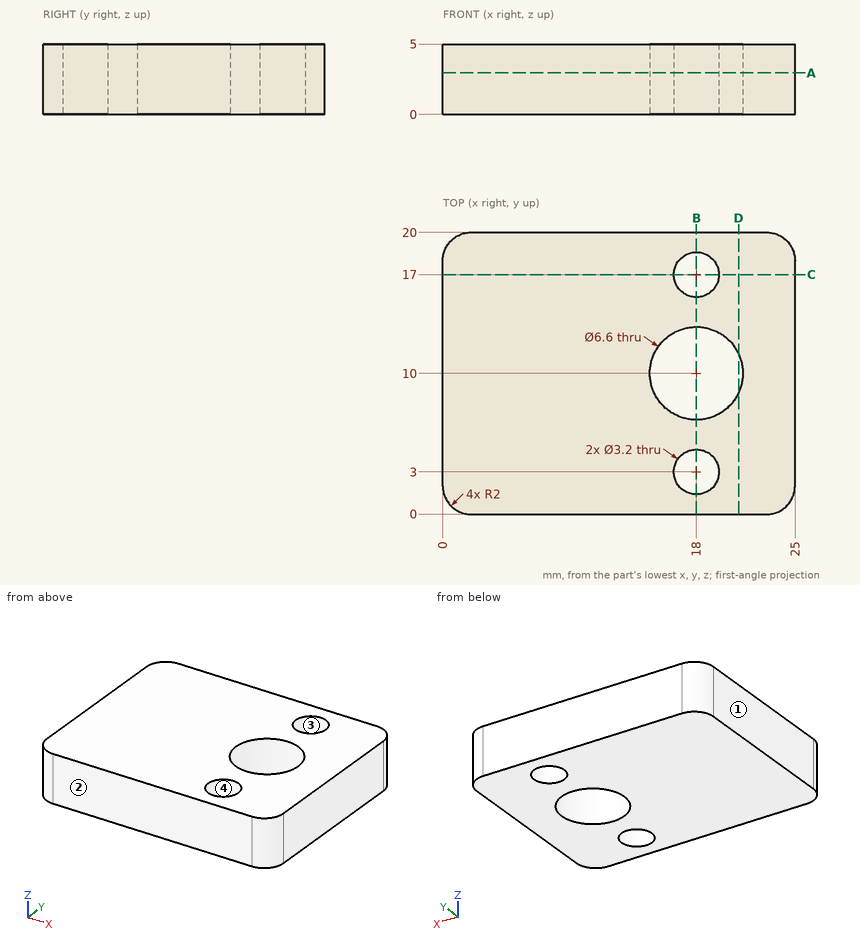
Part print with two shaded views. Sizes in mm from the minimum x, y, z corner. Round coordinates to 2 decimals unless told otherwise and drop trailing zeros. Order: outer loops, then holes, each group sorted by start corner. A loop starts at its lowest first (then second) coordinate and runs counter-clockwise, first axis right, second up. Notation, with made-up numbers: M 43,77.25 L 52,77.25 A32 cw 52,110.25 Z; hole C 36,17.5 d4. An arc over 180 degrees is marked long. Put each result on its own line as item: value. Start each with the question number.
1. Slice it at A-A on z = 2.95. List the corners of the cut face in (x, y), then the cut area to 3 significant figures.
2. Slice it at C-C on y = 17. List the corners of the cut face in (x, z).
3. Slice it at B-B on x = 18. List the corners of the cut face in (y, z).
4. Two-plate mould, pull along Y, no slides. Class the marked faces 1, 2, 3 and 4: +Y half, -Y half, draft (parallel to the pull), parting line (faces both ways), or undercut.
5. Slice it at D-D on x = 21. List the corners of the cut face in (y, z).
6. Drill centre lines: probe 1 along Y at (x, z) = (18, 2.1); probe 2 along Y at (x, z) = (19.25, 1.3); probe 3 along X at (y, z) = (16.25, 1.55). Where is each one in solid material? Low to high. Write a range as [from, to].
Findings:
1. outline: M 0,2 A2 ccw 2,0 L 23,0 A2 ccw 25,2 L 25,18 A2 ccw 23,20 L 2,20 A2 ccw 0,18 Z; hole C 18,10 d6.6; hole C 18,3 d3.2; hole C 18,17 d3.2
1. area: 446 mm2
2. outline: M 0,0 L 16.4,0 L 16.4,5 L 0,5 Z; M 19.6,0 L 25,0 L 25,5 L 19.6,5 Z
3. outline: M 0,0 L 1.4,0 L 1.4,5 L 0,5 Z; M 4.6,0 L 6.7,0 L 6.7,5 L 4.6,5 Z; M 13.3,0 L 15.4,0 L 15.4,5 L 13.3,5 Z; M 18.6,0 L 20,0 L 20,5 L 18.6,5 Z
4. face 1: draft
4. face 2: -Y half
4. face 3: undercut
4. face 4: undercut
5. outline: M 0,0 L 8.63,0 L 8.63,5 L 0,5 Z; M 11.37,0 L 20,0 L 20,5 L 11.37,5 Z
6. probe 1: [0, 1.4], [4.6, 6.7], [13.3, 15.4], [18.6, 20]
6. probe 2: [0, 2], [4, 6.95], [13.05, 16], [18, 20]
6. probe 3: [0, 16.59], [19.41, 25]
